Autodesk Inventor part; units mm, degrees
ref_plane "YZ Plane" through (0, 0, 0) normal (1, 0, 0) x (0, 1, 0)
ref_plane "XZ Plane" through (0, 0, 0) normal (0, 1, 0) x (-1, 0, 0)
ref_plane "XY Plane" through (0, 0, 0) normal (0, 0, 1) x (1, 0, 0)
sketch "Boceto1" plane through (0, 0, 0) normal (0, 0, 1) x (1, 0, 0)
  line L0 (0, 0) -> (76, 0)
  line L1 (76, 0) -> (76, 73)
  line L2 (76, 73) -> (73, 73)
  line L3 (73, 73) -> (73, 3)
  line L4 (73, 3) -> (3, 3)
  line L5 (3, 3) -> (3, 73)
  line L6 (3, 73) -> (0, 73)
  line L7 (0, 73) -> (0, 0)
extrude "Extrusión1" add sketch "Boceto1" against normal blind 50
sketch "Boceto2" plane through (76, 0, 0) normal (1, 0, 0) x (0, 0, -1)
  circle A0 centre (25, 49) radius 6.5
  circle A1 centre (20, 63) radius 2.5
  circle A2 centre (30, 63) radius 2.5
  circle A3 centre (20, 14.5) radius 2.5
  circle A4 centre (30, 14.5) radius 2.5
  point P0 (0, 0)
  point P1 (0, 73)
hole "Agujero1" at (76, 63, -20) at (76, 63, -30) at (76, 14.5, -20) at (76, 14.5, -30) direction (-1, 0, 0) diameter 5 end through all
hole "Agujero2" at (76, 49, -25) direction (-1, 0, 0) diameter 13 end through all
sketch "Boceto3" plane through (3, 3, 0) normal (0, 1, 0) x (1, 0, 0)
  circle A0 centre (35, 25) radius 4.5
  circle A1 centre (46.5, 31.75) radius 1.25
  circle A2 centre (46.5, 18.25) radius 1.25
  circle A3 centre (23.5, 31.75) radius 1.25
  circle A4 centre (23.5, 18.25) radius 1.25
hole "Agujero3" at (38, 3, -25) direction (0, -1, 0) diameter 9 end through all
hole "Agujero4" at (26.5, 3, -18.25) at (26.5, 3, -31.75) at (49.5, 3, -31.75) at (49.5, 3, -18.25) direction (0, -1, 0) diameter 2.5 end through all
fillet "Empalme1" radius 5 4 edges at (1.5, 73, 0) (1.5, 73, -50) (74.5, 73, 0) (74.5, 73, -50)
sketch "Boceto4" plane through (76, 0, 0) normal (1, 0, 0) x (0, 0, -1)
  circle A0 centre (25, 49) radius 6.5
  arc A1 (34.5, 44.5279) -> (15.5, 44.5279) centre (25, 49) ccw
  line L0 (25, 22) -> (34.5, 22)
  line L1 (34.5, 22) -> (34.5, 44.5279)
  line L2 (25, 22) -> (15.5, 22)
  line L3 (15.5, 22) -> (15.5, 44.5279)
  point P0 (0, 0)
  dimension "d68" = 9.5
  dimension "d69" = 9.5
extrude "Extrusión2" cut sketch "Boceto4" against normal blind 100 contours A0 | L1 L0 L2 L3 A1
properties part number "7"
Here's how the part is built. I have some questions about the finished solid (model axes, mm). A direction names the side the tool comes from. Coordinates: 2 decimals unless noted, no trailing zeros. Loops run counter-clockwise (first coordinate to the right, second up) from the corner with the lowest first, then second, coordinate; pieces in that order, holes last. Notation, with made-up numbers: (38, 63) - (77, 63) arc R11 ccw to (77, 78) - close; hole circle Ø11 at (-26.5, -25). An arc over 180 degrees is marked (long way). Return JSON: item names as keys, results as strings. Group by question number.
Item 1: On a 3-axis mill with a long thin cutter (end or side, diameter ignored), from which of +Z, -Z, +X, -X, +Y, -Y can I reach the whole of each face in a straight line? I mean faces 1 (the face through (42.39, 1.48, -25.98)), 2 (the face through (2, 22, -25)), 3 (the face through (73, 38, -36)). Say none if no direction works.
Item 2: If we section it at A-A on x = 49.5: Write out the boundary of the cut face in (y, z), and give its area (3 significant figures).
Item 3: I need wall thicknesses on line 1 (Z direction, x = 1, y = 63); line 2 (X direction, y = 28, z = -3); line 3 (Z direction, x = 74.1, y = 49). Which ranges of each line are inside material? Lowest first, please. Write a range as from..to.
Item 4: If we section it at D-D on z = -24: Write out the boundary of the cut face in (x, y).
Item 5: We'd pull the mould along Y, two halves only. Please class faces 4 (the face through (76, 36, -14)), 5 (the face through (2, 33, -34.5)), 6 (the face through (74, 71, -1)), 7 (the face through (37, 0, -19)): +Y half, -Y half, draft (parallel to the pull), parting line (faces both ways), or undercut.
Item 6: If we section it at B-B on y = 23.5: Write out the boundary of the cut face in (x, z), and give its area (3 significant figures).
Item 7: If we section it at C-C on y = 14.5: Write out the boundary of the cut face in (x, z), and give its area (3 significant figures).
Item 8: Will these pins go through, and if not, where does the flat tip stop? P1, Ø4.5, axis at y = 63, z = -30, coming from the +X side; P2, Ø2.5, axis at x = 2, y = 38.5, coming from the +Z side; P3, Ø8, axis at x = 53.5, z = -39.5, coming from the +Y side.
Calculated:
{
 "1": {"face 1": "+Y, -Y", "face 2": "+X, -X", "face 3": "+Z, -Z, +Y"},
 "2": {"outline": "(0, -50) - (3, -50) - (3, -33) - (0, -33) - close; (0, -30.5) - (3, -30.5) - (3, -19.5) - (0, -19.5) - close; (0, -17) - (3, -17) - (3, 0) - (0, 0) - close", "area": "135 mm^2"},
 "3": {"line 1": "z = -50..-32.5, -27.5..-22.5, -17.5..0", "line 2": "x = 0..3, 73..76", "line 3": "z = -50..-35.5, -14.5..0"},
 "4": {"outline": "(0, 0) - (33.61, 0) - (33.61, 3) - (3, 3) - (3, 22) - (0, 22) - close; (0, 59.45) - (3, 59.45) - (3, 73) - (0, 73) - close; (42.39, 0) - (76, 0) - (76, 22) - (73, 22) - (73, 3) - (42.39, 3) - close; (73, 59.45) - (76, 59.45) - (76, 73) - (73, 73) - close"},
 "5": {"face 4": "draft", "face 5": "undercut", "face 6": "+Y half", "face 7": "-Y half"},
 "6": {"outline": "(0, -50) - (3, -50) - (3, -34.5) - (0, -34.5) - close; (0, -15.5) - (3, -15.5) - (3, 0) - (0, 0) - close; (73, -50) - (76, -50) - (76, -34.5) - (73, -34.5) - close; (73, -15.5) - (76, -15.5) - (76, 0) - (73, 0) - close", "area": "186 mm^2"},
 "7": {"outline": "(0, -50) - (3, -50) - (3, -32.5) - (0, -32.5) - close; (0, -27.5) - (3, -27.5) - (3, -22.5) - (0, -22.5) - close; (0, -17.5) - (3, -17.5) - (3, 0) - (0, 0) - close; (73, -50) - (76, -50) - (76, -32.5) - (73, -32.5) - close; (73, -27.5) - (76, -27.5) - (76, -22.5) - (73, -22.5) - close; (73, -17.5) - (76, -17.5) - (76, 0) - (73, 0) - close", "area": "240 mm^2"},
 "8": {"P1": "passes through", "P2": "stops at z = 0", "P3": "stops at y = 3"}
}
